Print and shaded views of the part. All mm, measured from the part's lowest x, y and z. Round coordinates to 2 decimals unless told otherwise and drop trailing zeros. Loops run counter-clockwise (first coordinate to the right, second up) from the corner with the lowest first, then second, coordinate; pieces in that order, holes last. Notation, with made-up numbers: (72, 14.25) - (82, 14.25) arc R28 ccw to (82, 32.25) - close; hole circle Ø1 at (66, -32.5). An arc over 180 degrees is marked (long way). Use one line per item in the form item = value.
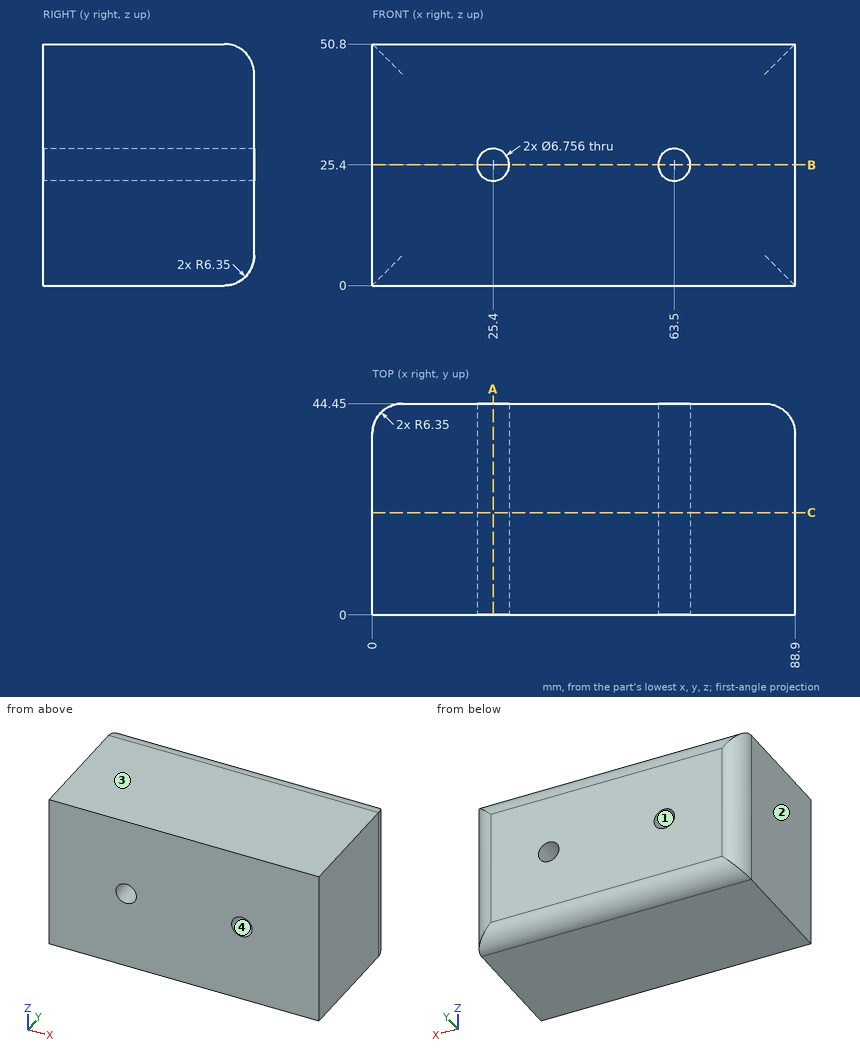
1. Cut at A-A, the plane x = 25.4. Give the cut face in (y, z), plus the area to 3 significant figures.
Geometry check:
outline = (0, 0) - (38.1, 0) arc R6.35 ccw to (44.45, 6.35) - (44.45, 22.02) - (0, 22.02) - close; (0, 28.78) - (44.45, 28.78) - (44.45, 44.45) arc R6.35 ccw to (38.1, 50.8) - (0, 50.8) - close
area = 1,940 mm^2
2. Wall check: probe 1 along Z at (x, y) = (25.4, 29.5); probe 2 along X at (y, z) = (16, 25) (1 decimal); probe 3 along Z at (x, y) = (63, 26). Give the ranges that are in metal, low to high.
Geometry check:
probe_1 = 0 to 22.02, 28.78 to 50.8
probe_2 = 0 to 22, 28.8 to 60.1, 66.9 to 88.9
probe_3 = 0 to 22.06, 28.74 to 50.8
3. Cut at B-B, the plane z = 25.4. Give the cut face in (x, y), plus the area to 3 significant figures.
Geometry check:
outline = (0, 0) - (22.02, 0) - (22.02, 44.45) - (6.35, 44.45) arc R6.35 ccw to (0, 38.1) - close; (28.78, 0) - (60.12, 0) - (60.12, 44.45) - (28.78, 44.45) - close; (66.88, 0) - (88.9, 0) - (88.9, 38.1) arc R6.35 ccw to (82.55, 44.45) - (66.88, 44.45) - close
area = 3,330 mm^2
4. Pull direction X, two halves, no side cores. Call the marked faces 1, 2, 3 and 4: +X half, -X half, draft (parallel to the pull), parting line (faces both ways), or undercut.
Geometry check:
face_1 = undercut
face_2 = -X half
face_3 = draft
face_4 = undercut
5. Cut at C-C, the plane y = 21.5. Give the cut face in (x, z), plus the area to 3 significant figures.
Geometry check:
outline = (0, 0) - (88.9, 0) - (88.9, 50.8) - (0, 50.8) - close; hole circle Ø6.76 at (25.4, 25.4); hole circle Ø6.76 at (63.5, 25.4)
area = 4,440 mm^2
